Geometry: final body of the model. Coordinates: model frame, mm. A direction names the side the tool comes from. Give positions to 0.01 mm unless a question says otherwise; leave off trailing zeros. Write each loop counter-clockwise with the first axis right and the second up, starting at its lowest first coordinate (ties: lowest second). Pieces come first, ordered by that corner, then holes. Notation, with made-up numbers: M 45,33 L 63,33 A28 ccw 63,62 Z; hole C -2.5,-39 d6. An arc over 180 degrees is marked long. Answer as a JSON object with one key per item and string values.
from build123d import *

# Parameters (mm, degrees)
BOSS_EXTRUDE1_DEPTH = 5
BOSS_EXTRUDE2_START = 5
SKETCH1_3_W         = 9.2
SKETCH1_3_H         = 6.5
BOSS_EXTRUDE2_DEPTH = 2
FILLET1_R           = 1


with BuildPart() as part:
    # Sketch1 → Boss-Extrude1 (new body)
    with BuildSketch(Plane.XY):
        Polygon((-12.95, 0), (-7.05, 0), (-7.05, 2), (-4.6, 2), (-4.6, 8.5), (4.6, 8.5), (4.6, 2), (7.05, 2), (7.05, 0), (12.95, 0), (12.95, 2), (12.95, 10), (-12.95, 10), (-12.95, 2), align=None)
        Polygon((-7.05, -3.8), (-12.95, -3.8), (-15.5, 0), (-4.5, 0), align=None)
        Polygon((4.5, 0), (15.5, 0), (12.95, -3.8), (7.05, -3.8), align=None)
    extrude(amount=BOSS_EXTRUDE1_DEPTH)

    # Sketch1<3> → Boss-Extrude2 (add)
    with BuildSketch(Plane.XY.offset(BOSS_EXTRUDE2_START)):
        with Locations((0, 5.25)):
            Rectangle(SKETCH1_3_W, SKETCH1_3_H)
        Polygon((-12.95, 0), (-7.05, 0), (-7.05, 2), (-4.6, 2), (-4.6, 8.5), (4.6, 8.5), (4.6, 2), (7.05, 2), (7.05, 0), (12.95, 0), (12.95, 2), (12.95, 10), (-12.95, 10), (-12.95, 2), align=None)
        Polygon((-7.05, -3.8), (-12.95, -3.8), (-15.5, 0), (-4.5, 0), align=None)
        Polygon((4.5, 0), (15.5, 0), (12.95, -3.8), (7.05, -3.8), align=None)
    extrude(amount=BOSS_EXTRUDE2_DEPTH)

    # Fillet1
    fillet1_edges = [part.edges().sort_by_distance(p)[0] for p in [
        (-4.5, 0, 3.5),
        (-7.05, -3.8, 3.5),
        (-12.95, -3.8, 3.5),
        (-15.5, 0, 3.5),
        (-12.95, 10, 3.5),
        (12.95, 10, 3.5),
        (15.5, 0, 3.5),
        (12.95, -3.8, 3.5),
        (7.05, -3.8, 3.5),
        (4.5, 0, 3.5),
        (4.6, 2, 2.5),
        (-4.6, 2, 2.5),
    ]]
    fillet(fillet1_edges, radius=FILLET1_R)


solid = part.part
1) Contact query for flat-ended pins moving along their axis: P1, Ø4, axis at y = 0, z = 5.5, coming from the +X side; P2, Ø0.5, axis at x = 13, z = 3, coming from the +Y side; P3, Ø2, axis at y = 6.5, z = 4, coming from the +X side; P4, Ø3.5, axis at x = -2, z = 4.5, coming from the -Y side. Output: stop coordinate, or through.
Geometry check:
{"P1": "stops at x = 14.62", "P2": "stops at y = 9.6", "P3": "stops at x = 12.95", "P4": "stops at y = 2"}
2) Line query: line 1 (X direction, y = 4.5, z = 1.25); line 2 (Y direction, x = 3.75, z = 2.5); line 3 (Z direction, x = 2.25, y = 4.25). Output: solid intervals per line, ascending. Write a range as from..to.
Geometry check:
{"line 1": "x = -12.95..-4.6, 4.6..12.95", "line 2": "y = 8.5..10", "line 3": "z = 5..7"}
3) Set-up query: faces 1 (the cylindrical face through (5.486, -0.543, 3.549)), 2 (the flat face through (-12.95, 5, 3)), 3 (the flat face through (-6.14, -2.445, 3.451)), 4 (the flat face through (4.6, 6, 2)). Return all of +Z, -Z, +X, -X, +Y, -Y with unobstructed straight access to the full face (end or side cutting, diameter ignored); none if empty.
Geometry check:
{"face 1": "+Z, -Z", "face 2": "+Z, -Z, -X, +Y", "face 3": "+Z, -Z, -Y", "face 4": "-Z, -Y"}
4) Pull-direction query (Y, two-part tool) for faces 5 (the cylindrical face through (12.649, 9.715, 3.549)), 6 (the cylindrical face through (-5.5, -0.52, 3.55)), 7 (the flat face through (-10, -3.8, 3)), 8 (the flat face through (6, 3, 0)); classes: pulls with the +Y half, pulls with the -Y half, needs draft (parallel to the pull), parting line crosses it, or undercut.
Geometry check:
{"face 5": "pulls with the +Y half", "face 6": "undercut", "face 7": "pulls with the -Y half", "face 8": "needs draft"}
5) Cut plane D-D on x = 0.5. Return loops of the section in (y, z), and give its area (3 significant figures).
Geometry check:
{"outline": "M 2,5 L 8.5,5 L 8.5,0 L 10,0 L 10,7 L 2,7 Z", "area": "23.5 mm2"}
6) Cut plane C-C on y = 7.5. Return loops of the section in (x, z), and give its area (3 significant figures).
Geometry check:
{"outline": "M -12.95,0 L -4.6,0 L -4.6,5 L 4.6,5 L 4.6,0 L 12.95,0 L 12.95,7 L -12.95,7 Z", "area": "135 mm2"}
7) Cut plane A-A on y = 1. Return loops of the section in (x, z).
Geometry check:
{"outline": "M -12.95,0 L -7.05,0 L -7.05,7 L -12.95,7 Z; M 7.05,0 L 12.95,0 L 12.95,7 L 7.05,7 Z"}
